Model file for the job. Use its own axes, mm. Face numbers are marked on the shaded views. A direction names the side the tool comes from. Round coordinates to 2 decimals unless told otherwise and drop trailing zeros. Loops run counter-clockwise (first coordinate to the right, second up) from the corner with the lowest first, then second, coordinate; pieces in that order, holes last. Notation, with made-up numbers: M 3,54 L 37,54 A27 ccw 37,74 Z; hole C 66.5,14.25 d4. An arc over 180 degrees is marked long. Use a Markdown table: item, result. Add a question column.
Item 1: Saw through at A-A on z = 30. Write the cut outline in (x, y), then the cut area to 3 significant figures.
Item 2: Saw through at C-C on x = 21.5. Write the cut outline in (y, z).
Item 3: Saw through at D-D on y = 20. Write the cut outline in (x, z), then the cut area to 3 significant figures.
Item 4: Pin check, flat tips, straight feed: P1, Ø10, axis at x = 12, z = 8, coming from the +Y side; P2, Ø5, axis at y = 14, z = 18.5, coming from the +X side. Stop position of each tip, or through.
Item 5: Saw through at B-B on y = 25. Write the cut outline in (x, z), then the cut area to 3 significant figures.
Item 6: Wall check: L1, parallel to Y at x = 2.55, z = 15.15; L2, parallel to Y at x = 8.5, z = 33. Give the ranges that are in metal, low to high. Write a range as from..to.
Item 7: Tool access for the marked faces 1 and 2: list every direction of +Z, -Z, +X, -X, +Y, -Y with a clear straight run to the whole face (end or side of a thin tool).
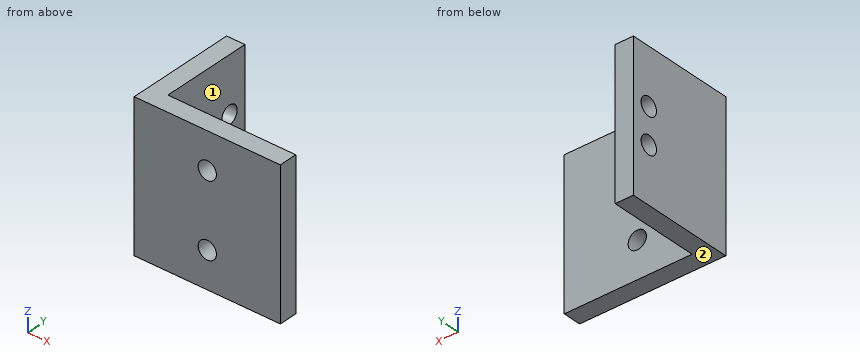
```python
from build123d import *

# Parameters (mm, degrees)
BOSS_EXTRUDE1_DEPTH = 40
SKETCH2_R           = 2.5
CUT_EXTRUDE1_DEPTH  = 40
SKETCH3_R           = 2.5
CUT_EXTRUDE2_DEPTH  = 40


with BuildPart() as part:
    # Sketch1 → Boss-Extrude1 (new body)
    with BuildSketch(Plane.XY):
        Polygon((0, 0), (0, 30), (5, 30), (5, 5), (40, 5), (40, 0), align=None)
    extrude(amount=BOSS_EXTRUDE1_DEPTH)

    # Sketch2 → Cut-Extrude1 (cut)
    with BuildSketch(Plane.ZY):
        with Locations((24.85, 25)):
            Circle(SKETCH2_R)
        with Locations((15.15, 25)):
            Circle(SKETCH2_R)
    extrude(amount=-CUT_EXTRUDE1_DEPTH, mode=Mode.SUBTRACT)

    # Sketch3 → Cut-Extrude2 (cut)
    with BuildSketch(Plane.XZ):
        with Locations((20, 30)):
            Circle(SKETCH3_R)
        with Locations((20, 10)):
            Circle(SKETCH3_R)
    extrude(amount=-CUT_EXTRUDE2_DEPTH, mode=Mode.SUBTRACT)


solid = part.part
```
Entries:
| question | item | result |
|---|---|---|
| 1 | outline | M 0,0 L 17.5,0 L 17.5,5 L 5,5 L 5,30 L 0,30 Z; M 22.5,0 L 40,0 L 40,5 L 22.5,5 Z |
| 1 | area | 300 mm2 |
| 2 | outline | M 0,0 L 5,0 L 5,8 L 0,8 Z; M 0,12 L 5,12 L 5,28 L 0,28 Z; M 0,32 L 5,32 L 5,40 L 0,40 Z |
| 3 | outline | M 0,0 L 5,0 L 5,40 L 0,40 Z |
| 3 | area | 200 mm2 |
| 4 | P1 | y = 5 |
| 4 | P2 | x = 5 |
| 5 | outline | M 0,0 L 5,0 L 5,12.65 L 0,12.65 Z; M 0,17.65 L 5,17.65 L 5,22.35 L 0,22.35 Z; M 0,27.35 L 5,27.35 L 5,40 L 0,40 Z |
| 5 | area | 150 mm2 |
| 6 | L1 | 0..22.5, 27.5..30 |
| 6 | L2 | 0..5 |
| 7 | face 1 | +Z, -Z, +X, +Y |
| 7 | face 2 | -Z, +X, -X, +Y, -Y |
